Work out the finished part from the listing and answer in its coordinate system (mm). Face numbers are marked on the shaded views. Give positions to 0.01 mm unless a question says otherwise; leave off trailing zeros. Order: outer loops, then holes, each group sorted by start corner. A loop starts at its lowest first (then second) coordinate and runs counter-clockwise, first axis right, second up.
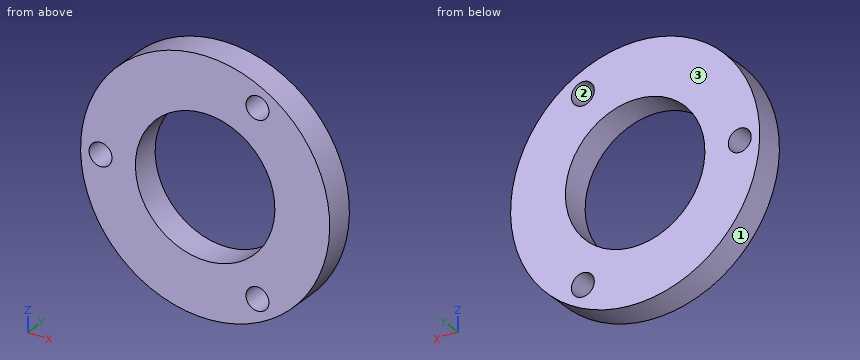
```python
from build123d import *

# Parameters (mm, degrees)
SKETCH1_R           = 12.5
SKETCH1_R_2         = 7
BOSS_EXTRUDE1_DEPTH = 3
CUT_EXTRUDE1_REACH  = 19.93
SKETCH3_R           = 1.15


with BuildPart() as part:
    # Sketch1 → Boss-Extrude1 (new body)
    with BuildSketch(Plane(origin=(0, 0, 0), x_dir=(1, 0, 0), z_dir=(0, 1, 0))):
        with Locations(Location((0, 0, 0), (0, 0, 270))):
            Circle(SKETCH1_R)
        with Locations(Location((0, 0, 0), (0, 0, 270))):
            Circle(SKETCH1_R_2, mode=Mode.SUBTRACT)
    extrude(amount=BOSS_EXTRUDE1_DEPTH)

    # Sketch3 → Cut-Extrude1 (cut, up to next)
    with BuildSketch(Plane(origin=(0, 3, 0), x_dir=(1, 0, 0), z_dir=(0, 1, 0)), mode=Mode.PRIVATE) as cut_extrude1_sk1:
        with Locations(Location((-10.5, 0, 0), (0, 0, 270))):
            Circle(SKETCH3_R)
    cut_extrude1_tool1 = extrude(cut_extrude1_sk1.sketch, amount=-CUT_EXTRUDE1_REACH, mode=Mode.PRIVATE) & part.part
    # Sketch3 → Cut-Extrude1 (cut, up to next)
    with BuildSketch(Plane(origin=(0, 3, 0), x_dir=(1, 0, 0), z_dir=(0, 1, 0)), mode=Mode.PRIVATE) as cut_extrude1_sk2:
        with Locations(Location((5.25, 9.09326674, 0), (0, 0, 270))):
            Circle(SKETCH3_R)
    cut_extrude1_tool2 = extrude(cut_extrude1_sk2.sketch, amount=-CUT_EXTRUDE1_REACH, mode=Mode.PRIVATE) & part.part
    # Sketch3 → Cut-Extrude1 (cut, up to next)
    with BuildSketch(Plane(origin=(0, 3, 0), x_dir=(1, 0, 0), z_dir=(0, 1, 0)), mode=Mode.PRIVATE) as cut_extrude1_sk3:
        with Locations(Location((5.25, -9.09326674, 0), (0, 0, 270))):
            Circle(SKETCH3_R)
    cut_extrude1_tool3 = extrude(cut_extrude1_sk3.sketch, amount=-CUT_EXTRUDE1_REACH, mode=Mode.PRIVATE) & part.part
    add(cut_extrude1_tool1.solids().sort_by_distance((-10.5, 3, 0))[0], mode=Mode.SUBTRACT)
    add(cut_extrude1_tool2.solids().sort_by_distance((5.25, 3, -9.093267))[0], mode=Mode.SUBTRACT)
    add(cut_extrude1_tool3.solids().sort_by_distance((5.25, 3, 9.093267))[0], mode=Mode.SUBTRACT)


solid = part.part
```
1. The part is cut by section A-A (x = 0). Write down the section's boundary in (y, z).
Findings below:
outline: (0, -12.5) - (3, -12.5) - (3, -7) - (0, -7) - close; (0, 7) - (3, 7) - (3, 12.5) - (0, 12.5) - close
2. The part is cut by section B-B (z = 0). Write down the section's boundary in (x, y).
Findings below:
outline: (-12.5, 0) - (-11.65, 0) - (-11.65, 3) - (-12.5, 3) - close; (-9.35, 0) - (-7, 0) - (-7, 3) - (-9.35, 3) - close; (7, 0) - (12.5, 0) - (12.5, 3) - (7, 3) - close
3. The part is cut by section D-D (x = 5.25). Write down the section's boundary in (y, z), then the cut area to 3 significant figures.
Findings below:
outline: (0, -11.34) - (3, -11.34) - (3, -10.24) - (0, -10.24) - close; (0, -7.94) - (3, -7.94) - (3, -4.63) - (0, -4.63) - close; (0, 4.63) - (3, 4.63) - (3, 7.94) - (0, 7.94) - close; (0, 10.24) - (3, 10.24) - (3, 11.34) - (0, 11.34) - close
area: 26.5 mm2
4. Straight lines are drawn through the part: probe 1 along X at (y, z) = (0.6, 0); probe 2 along Z at (x, y) = (6.25, 1); probe 3 along X at (y, z) = (1.65, 1). For each, find the intervals that lie inside material, in ascending order.
Findings below:
probe 1: x = -12.5 to -11.65, -9.35 to -7, 7 to 12.5
probe 2: z = -10.83 to -9.66, -8.53 to -3.15, 3.15 to 8.53, 9.66 to 10.83
probe 3: x = -12.46 to -11.07, -9.93 to -6.93, 6.93 to 12.46
5. The part is cut by section C-C (y = 1.25). Write down the section's boundary in (x, z), then the cut area to 3 significant figures.
Findings below:
outline: circle Ø25 at (0, 0); hole circle Ø2.3 at (-10.5, 0); hole circle Ø14 at (0, 0); hole circle Ø2.3 at (5.25, -9.09); hole circle Ø2.3 at (5.25, 9.09)
area: 324 mm2
6. The mould has two halves that part along X. Classify the marked faces 1, 2 and 3: pulls with the +X half, pulls with the -X half, needs draft (parallel to the pull), parting line crosses it, or undercut.
Findings below:
face 1: parting line crosses it
face 2: undercut
face 3: needs draft
